Model file for the job. Use its own axes, mm. A direction names the side the tool comes from. Give positions to 0.01 mm unless a question says otherwise; leave off trailing zeros. Loops run counter-clockwise (first coordinate to the right, second up) from the corner with the lowest first, then second, coordinate; pieces in that order, holes last. Notation, with made-up numbers: (-3.75, -17.75) -> (45.25, -17.75) arc R22 cw to (45.25, -8.75) -> close; hole circle Ø3 at (-9, 88). An arc over 180 degrees is marked (long way). Use CSV: the item, a comma, the result in double quotes. Start each with the question number.
(1) 3-axis set-ups, long thin cutter, end or side, ignore diameter. For faces 1 (the flat face through (9.067, 33.741, 7.535)), 2 (the flat face through (-1, 30, 10)): which of +Z, -Z, +X, -X, +Y, -Y reach the whole face in a straight line?
(2) Cut at A-A on z = 9. State how many separate pieces and enclosed holes the cut face has, then the cut area to 3 significant figures.
(3) Pull direction X, two halves, no side cores. Call faces 3 (the flat face through (50, 30, 5)), 4 (the cylindrical face through (26.526, 34.224, 7.465)), 5 (the flat face through (-1, 30, 0)): pulls with the +X half, pulls with the -X half, needs draft (parallel to the pull), parting line crosses it, or undercut.
(4) Drill centre lines: probe 1 along Y at (x, z) = (-17.5, 5.5); probe 2 along X at (y, z) = (26.5, 9.25); probe 3 along X at (y, z) = (43, 9). Where is each one in solid material? Low to high.
(5) Cut at B-B on y = 24. Write the cut outline in (x, z), then the cut area to 3 significant figures.
from build123d import *

# Parameters (mm, degrees)
SKETCH3_W           = 100
SKETCH3_H           = 60
BOSS_EXTRUDE3_DEPTH = 10
CUT_EXTRUDE1_START  = 10
CUT_EXTRUDE1_DEPTH  = 5
FILLET1_R           = 1


with BuildPart() as part:
    # Sketch3 → Boss-Extrude3 (new body)
    with BuildSketch(Plane.XY):
        with Locations((0, 30)):
            Rectangle(SKETCH3_W, SKETCH3_H)
    extrude(amount=BOSS_EXTRUDE3_DEPTH)

    # Sketch1<2> → Cut-Extrude1 (cut)
    with BuildSketch(Plane.XY.offset(CUT_EXTRUDE1_START)):
        Polygon((-21.712736005, 45), (-4.789659082, 45), (-4.789659082, 41.923076923), (-19.020428312, 41.923076923), (-19.020428312, 32.692307692), (-4.789659082, 32.692307692), (-4.789659082, 29.615384615), (-19.020428312, 29.615384615), (-19.020428312, 18.076923077), (-4.789659082, 18.076923077), (-4.789659082, 15), (-21.712736005, 15), align=None)
        Polygon((-0.943505235, 15), (3.016831303, 45), (3.401446688, 45), (15.787263995, 20.384615385), (28.143033226, 45), (28.533658226, 45), (32.518033226, 15), (29.813706303, 15), (26.941110149, 36.586538462), (16.111783226, 15), (15.504812072, 15), (4.633417841, 36.634615385), (1.766831303, 15), align=None)
    extrude(amount=-CUT_EXTRUDE1_DEPTH, mode=Mode.SUBTRACT)

    # Fillet1
    fillet1_edges = [part.edges().sort_by_distance(p)[0] for p in [
        (-4.789659082, 15, 7.5),
        (-21.712736005, 15, 7.5),
        (-21.712736005, 45, 7.5),
        (-4.789659082, 45, 7.5),
        (-4.789659082, 41.923076923, 7.5),
        (-19.020428312, 41.923076923, 7.5),
        (-19.020428312, 32.692307692, 7.5),
        (-4.789659082, 32.692307692, 7.5),
        (-4.789659082, 29.615384615, 7.5),
        (-19.020428312, 29.615384615, 7.5),
        (-19.020428312, 18.076923077, 7.5),
        (-4.789659082, 18.076923077, 7.5),
        (15.787263995, 20.384615385, 7.5),
        (32.518033226, 15, 7.5),
        (29.813706303, 15, 7.5),
        (26.941110149, 36.586538462, 7.5),
        (4.633417841, 36.634615385, 7.5),
        (1.766831303, 15, 7.5),
        (-0.943505235, 15, 7.5),
    ]]
    fillet(fillet1_edges, radius=FILLET1_R)


solid = part.part
Check result:
1,face 1,"+Z"
1,face 2,"+Z, +X, -X, +Y, -Y"
2,separate pieces,"1"
2,enclosed holes,"2"
2,area,"5,500 mm²"
3,face 3,"pulls with the +X half"
3,face 4,"undercut"
3,face 5,"needs draft"
4,probe 1,"0 to 15, 18.08 to 29.62, 32.69 to 41.92, 45 to 60"
4,probe 2,"-50 to -21.71, -19.02 to 0.57, 3.29 to 9.73, 12.71 to 18.86, 21.88 to 28.28, 30.99 to 50"
4,probe 3,"-50 to -21.71, -4.79 to 2.75, 4.41 to 27.14, 28.8 to 50"
5,outline,"(-50, 0) -> (50, 0) -> (50, 10) -> (31.32, 10) -> (31.32, 5) -> (28.62, 5) -> (28.62, 10) -> (20.63, 10) -> (20.63, 5) -> (17.6, 5) -> (17.6, 10) -> (13.97, 10) -> (13.97, 5) -> (10.98, 5) -> (10.98, 10) -> (2.96, 10) -> (2.96, 5) -> (0.24, 5) -> (0.24, 10) -> (-19.02, 10) -> (-19.02, 5) -> (-21.71, 5) -> (-21.71, 10) -> (-50, 10) -> close"
5,area,"929 mm²"
